Could you check a few things on this model? Use its own coordinates, in mm. Face numbers are marked on the shaded views. A direction names the side the tool comes from. Give positions to 0.01 mm unless a question says otherwise; leave off trailing zeros. Write each loop counter-clockwise with the first axis right and the second up, starting at its lowest first coordinate (ties: lowest second). Pieces come first, ordered by that corner, then holes. Notation, with made-up numbers: M 28.25,-19 L 34.25,-19 A18 cw 34.25,-12 Z; hole C -11.75,-23.5 d11. An arc over 180 degrees is marked long. Use one line per item in the form item = value.
from build123d import *

# Parameters (mm, degrees)
HIERRO_ANGULAR_2_X_2_X_0_125_1_DEPTH = 300


with BuildPart() as part:
    # Sketch11 → Hierro angular 2 X 2 X 0.125(1) (new body)
    with BuildSketch(Plane(origin=(0, -150, 0), x_dir=(-1, 0, 0), z_dir=(0, 1, 0))):
        with BuildLine():
            Line((0, 0), (0, 50.8))
            Line((0, 50.8), (0.00508, 50.8))
            ThreePointArc((0.00508, 50.8), (2.246551928, 49.871551928), (3.175, 47.63008))
            Line((3.175, 47.63008), (3.175, 7.9375))
            ThreePointArc((3.175, 7.9375), (4.569903955, 4.569903955), (7.9375, 3.175))
            Line((7.9375, 3.175), (47.63008, 3.175))
            ThreePointArc((47.63008, 3.175), (49.871551928, 2.246551928), (50.8, 0.00508))
            Line((50.8, 0.00508), (50.8, 0))
            Line((50.8, 0), (0, 0))
        make_face()
    extrude(amount=HIERRO_ANGULAR_2_X_2_X_0_125_1_DEPTH)


solid = part.part
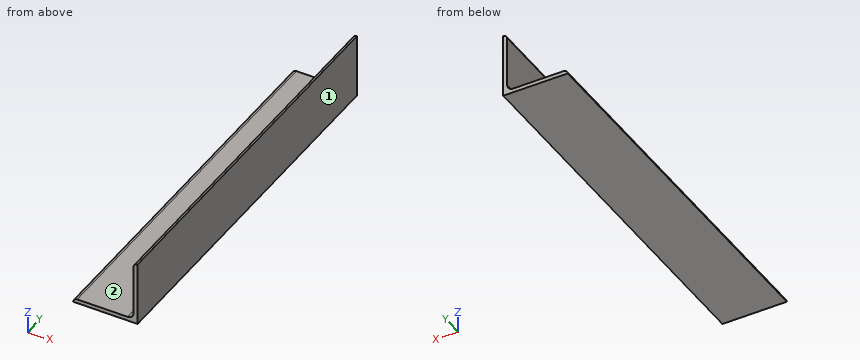
1) If I drill on L1, parallel to X at y = 39.5, z = 29 (3 decimals); L2, parallel to Z at x = -43, y = 63 (3 decimals); L3, parallel to X at y = -26, z = 2, over which ranges is the centre line in solid material (lowest first)?
Checked values:
L1 = -3.175 to 0
L2 = 0 to 3.175
L3 = -50.09 to 0
2) For pin 1 Ø10 at (x, y) = (-41.5, -78.5) entering from +Z (3 decimals); pin 2 Ø12 at (y, z) = (19, 35) entering from -X (3 decimals), each with a flat end and sliding along its axis, tell me the tip position at first contact or that it passes through.
Checked values:
pin_1 = 3.175
pin_2 = -3.175
3) I want a section at B-B, the plane x = -38.5. Please give me the cut outline in (y, z) (3 decimals), plus the area to 4 significant figures.
Checked values:
outline = M -150,0 L 150,0 L 150,3.175 L -150,3.175 Z
area = 952.5 mm2
4) I want a section at C-C, the plane z = 30.5. Please give me the cut outline in (x, y) (3 decimals).
Checked values:
outline = M -3.175,-150 L 0,-150 L 0,150 L -3.175,150 Z
5) For the marked faces 1 and 2, which set-ups out of +Z, -Z, +X, -X, +Y, -Y let a thin tool reach every point of the face, with its end or its side?
Checked values:
face_1 = +Z, -Z, +X, +Y, -Y
face_2 = +Z, -X, +Y, -Y
